```python
from build123d import *

# Parameters (mm, degrees)
PAD_DEPTH         = 28
SKETCH001_R       = 1.8
POCKET_DEPTH      = 6.151
POCKET_DEPTH_BACK = -6.151
FILLET_R          = 3
FILLET001_R       = 1


with BuildPart() as part:
    # Sketch → Pad (new body)
    with BuildSketch(Plane.XY):
        with BuildLine():
            ThreePointArc((3.487119, 0), (0, 6.4), (-3.487119, 0))
            Line((-3.487119, -23.9), (-3.487119, 0))
            Line((-5.487119, -23.9), (-3.487119, -23.9))
            Line((-5.487119, -0.527413), (-5.487119, -23.9))
            ThreePointArc((5.487119, -0.527413), (0, 8.4), (-5.487119, -0.527413))
            Line((5.487119, -23.9), (5.487119, -0.527413))
            Line((3.487119, -23.9), (5.487119, -23.9))
            Line((3.487119, 0), (3.487119, -23.9))
        make_face()
    extrude(amount=PAD_DEPTH)

    # Sketch001 → Pocket (cut, two sides)
    with BuildSketch(Plane.YZ) as pocket_sk:
        with Locations((-11.9, 14)):
            Circle(SKETCH001_R)
    extrude(amount=-POCKET_DEPTH, mode=Mode.SUBTRACT)
    extrude(pocket_sk.sketch, amount=-POCKET_DEPTH_BACK, mode=Mode.SUBTRACT)

    # Fillet
    fillet_edges = [part.edges().sort_by_distance(p)[0] for p in [
        (3.487119, 0, 14),
        (-3.487119, 0, 14),
        (5.487119, -0.527413, 14),
        (-5.487119, -0.527413, 14),
    ]]
    fillet(fillet_edges, radius=FILLET_R)

    # Fillet001
    fillet001_edges = [part.edges().sort_by_distance(p)[0] for p in [
        (4.487119, -23.9, 28),
        (-4.487119, -23.9, 28),
        (-4.487119, -23.9, 0),
        (4.487119, -23.9, 0),
    ]]
    fillet(fillet001_edges, radius=FILLET001_R)


solid = part.part
```
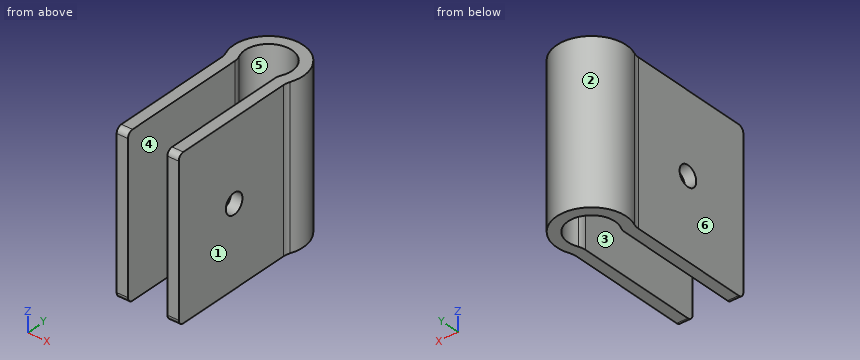
Input: part model. Units: mm. Frame: model coordinates. Face numbers are marked on the shaded views. A direction names the side the tool comes from. Give positions to 0.01 mm unless a question says otherwise; leave off trailing zeros. Order: outer loops, then holes, each group sorted by start corner. A loop starts at its lowest first (then second) coordinate and runs counter-clockwise, first axis right, second up.
1. Cut plane A-A (z = 14). Return loops of the section in (x, y).
Computed:
outline: (-5.7, -0.05) arc R3 cw to (-5.49, -1.17) - (-5.49, -10.1) - (-3.49, -10.1) - (-3.49, -0.76) arc R3 ccw to (-3.77, 0.5) arc R4.15 cw (long way) to (3.77, 0.5) arc R3 ccw to (3.49, -0.76) - (3.49, -10.1) - (5.49, -10.1) - (5.49, -1.17) arc R3 cw to (5.7, -0.05) arc R6.15 ccw (long way) to start; (-5.49, -23.9) - (-3.49, -23.9) - (-3.49, -13.7) - (-5.49, -13.7) - close; (3.49, -23.9) - (5.49, -23.9) - (5.49, -13.7) - (3.49, -13.7) - close
2. Pin query (flat end, axial travel): pin 1 Ø2 at (y, z) = (-11.9, 14) entering from -X; pin 2 Ø3 at (y, z) = (-7, 24.5) entering from +X; pin 3 Ø11.5 at (y, z) = (-9.5, 9) entering from -X. Return the tip coordinate at first contact, or that it passes through.
Computed:
pin 1: passes through
pin 2: stops at x = 5.49
pin 3: stops at x = -5.49
3. Cut plane D-D (z = 21.75). Return loops of the section in (x, y).
Computed:
outline: (-5.7, -0.05) arc R3 cw to (-5.49, -1.17) - (-5.49, -23.9) - (-3.49, -23.9) - (-3.49, -0.76) arc R3 ccw to (-3.77, 0.5) arc R4.15 cw (long way) to (3.77, 0.5) arc R3 ccw to (3.49, -0.76) - (3.49, -23.9) - (5.49, -23.9) - (5.49, -1.17) arc R3 cw to (5.7, -0.05) arc R6.15 ccw (long way) to start
4. Cut plane B-B (y = 2.25). Return loops of the section in (x, z).
Computed:
outline: (-6.15, 0) - (-4.15, 0) - (-4.15, 28) - (-6.15, 28) - close; (4.15, 0) - (6.15, 0) - (6.15, 28) - (4.15, 28) - close
5. Cut plane C-C (y = -11.9). Return loops of the section in (x, z).
Computed:
outline: (-5.49, 0) - (-3.49, 0) - (-3.49, 12.2) - (-5.49, 12.2) - close; (-5.49, 15.8) - (-3.49, 15.8) - (-3.49, 28) - (-5.49, 28) - close; (3.49, 0) - (5.49, 0) - (5.49, 12.2) - (3.49, 12.2) - close; (3.49, 15.8) - (5.49, 15.8) - (5.49, 28) - (3.49, 28) - close
6. Draft query along X for the marked faces 1, 2 and 3. Return one class per face: released by +X, released by -X, zero draft, split by the parting line, or undercut.
Computed:
face 1: released by +X
face 2: split by the parting line
face 3: undercut
7. Line query: probe 1 along X at (y, z) = (-17.5, 16); probe 2 along Z at (x, y) = (-4, -11.9); probe 3 along X at (y, z) = (2.25, 7). Output: solid intervals per line, ascending.
Computed:
probe 1: x = -5.49 to -3.49, 3.49 to 5.49
probe 2: z = 0 to 12.2, 15.8 to 28
probe 3: x = -6.15 to -4.15, 4.15 to 6.15
8. Set-up query: the marked faces 4, 5 and 6. Return all of +Z, -Z, +X, -X, +Y, -Y with unobstructed straight access to the full face (end or side cutting, diameter ignored); none if empty.
Computed:
face 4: +Z, -Z, -Y
face 5: +Z, -Z
face 6: +Z, -Z, -X, -Y
